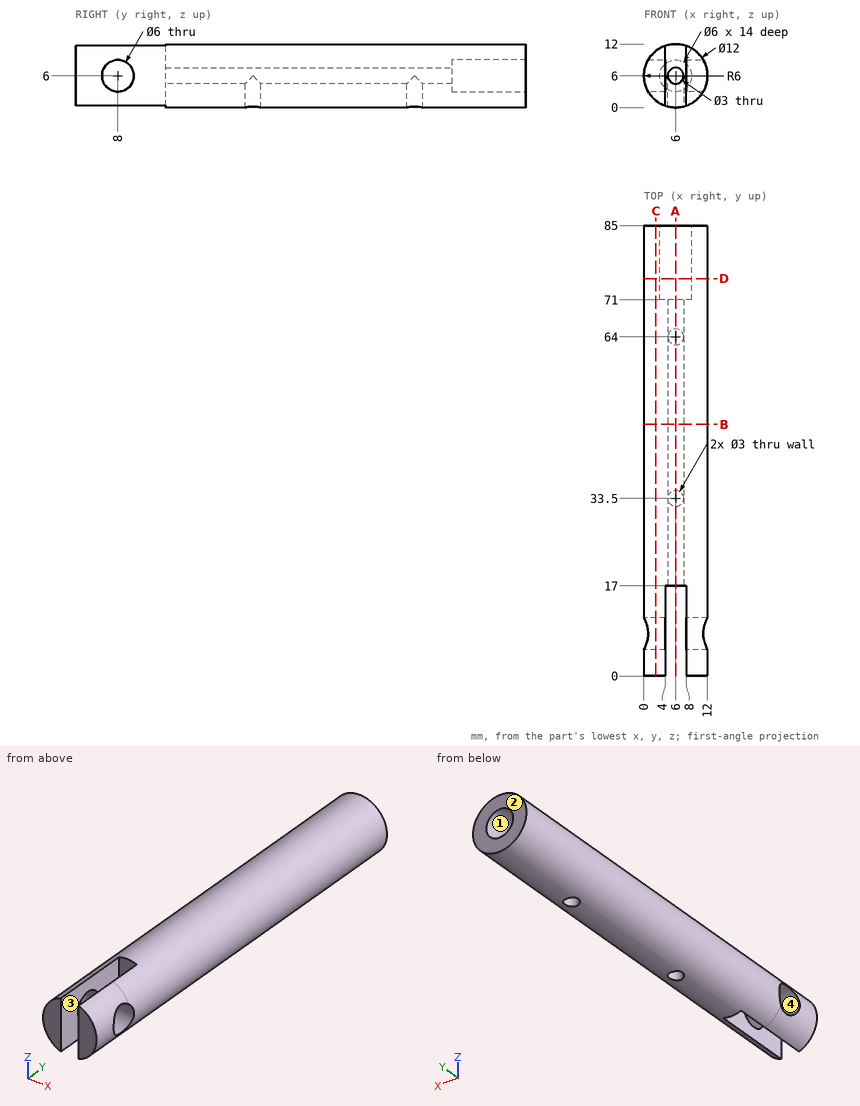
Study the drawing (mm; zero at the part's minimum x, y, z) and answer. A direction names the side the tool comes from. Coordinates: 2 decimals unless noted, no trailing zeros. Write each loop counter-clockwise with the first axis right and the second up, starting at its lowest first coordinate (ties: lowest second). Pieces come first, ordered by that corner, then holes. Notation, with made-up numbers: M 75,-23.5 L 133,-23.5 A32 cw 133,5.5 Z; hole C 57,44.5 d2. An arc over 180 degrees is marked long. Use one line per item in the form item = value.
Item 1: For the marked faces 3 and 4, determine the directions among +Z, -Z, +X, -X, +Y, -Y from which every point of the face is accessible in a straight line to the end or side of a thin tool.
Model answer:
face_3 = +Z, -Z, -Y
face_4 = +X, -X
Item 2: The mould has two halves that part along X. Classify the marked faces 1 and 2: released by +X, released by -X, zero draft, split by the parting line, or undercut.
Model answer:
face_1 = undercut
face_2 = zero draft
Item 3: Find section A-A, the plane x = 6. Give the vertices of the cut face in (y, z), plus the area to 3 significant figures.
Model answer:
outline = M 17,0 L 32,0 L 32,4.5 L 17,4.5 Z; M 17,7.5 L 71,7.5 L 71,9 L 85,9 L 85,12 L 17,12 Z; M 35,0 L 62.5,0 L 62.5,4.5 L 35,4.5 Z; M 65.5,0 L 85,0 L 85,3 L 71,3 L 71,4.5 L 65.5,4.5 Z
area = 543 mm2
Item 4: Find section D-D, the plane y = 75. Give the vertices of the cut face in (x, z).
Model answer:
outline = C 6,6 d12; hole C 6,6 d6
Item 5: Find section C-C, the plane x = 2.25. Give the vertices of the cut face in (y, z).
Model answer:
outline = M 0,1.32 L 85,1.32 L 85,10.68 L 0,10.68 Z; hole C 8,6 d6
Item 6: Find the intervals of material crossed by probe 1 along X at (y, z) = (78.25, 6); probe 2 along X at (y, z) = (14, 9.5); probe 3 along Z at (x, y) = (6.25, 39), in increasing order.
Model answer:
probe_1 = 0 to 3, 9 to 12
probe_2 = 1.13 to 4, 8 to 10.87
probe_3 = 0.01 to 4.52, 7.48 to 11.99
Item 7: Find section B-B, the plane y = 47.5. Give the vertices of the cut face in (x, z).
Model answer:
outline = C 6,6 d12; hole C 6,6 d3
Item 8: Given P1, Ø1.2, axis at x = 6, z = 7.5, coming from the -Y side; P2, Ø5, axis at x = 6, z = 6, coming from the +Y side; P3, Ø4, axis at x = 2.5, y = 71.5, coming from the -Z side, each flat-ended and moving along its own axis, determine where each tip first touches the part or whether it passes through.
Model answer:
P1 = 17
P2 = 71
P3 = 0.19
